Design review of the part built by this model. Coordinates are the model's own, in mm. Give positions to 0.01 mm unless a question says otherwise; leave off trailing zeros. Loops run counter-clockwise (first coordinate to the right, second up) from the corner with the lowest first, then second, coordinate; pieces in that order, holes last. Notation, with made-up numbers: (-20.5, 35.25) -> (-10.5, 35.25) arc R5 ccw to (-10.5, 40.25) -> close; hole circle Ø2 at (37, 73). An arc over 180 degrees is marked (long way). Use a Markdown table: item, result. Add a question column.
1. Draft analysis for pull direction X (two halves, no side actions). For faces 1 (the flat face through (0, 50.2, 2)), 2 (the flat face through (-1.1, -32.5, 0)), state which applies: pulls with the +X half, pulls with the -X half, needs draft (parallel to the pull), parting line crosses it, or undercut.
2. Add section B-B (x = 0). State the section outline as (y, z) points.
3. Add section D-D (x = 36). State the section outline as (y, z) points, and give its area (3 significant figures).
4. Add section C-C (z = 2.75). State the section outline as (x, y) points, and give its area (3 significant figures).
5. For pin 1 Ø1.5 at (y, z) = (62, 3.5) entering from -X; pin 2 Ø1.5 at (x, z) = (-57, 1.5) entering from -Y; pin 3 Ø1.5 at (x, z) = (13, 1.5) entering from +Y, all flat-tipped, find the tip position at first contact; note any pin that passes through.
6. To check wall thickness, follow line 1 (Y direction, x = -0.5, z = 3.95); line 2 (Y direction, x = -24.5, z = 2.35); line 3 (Y direction, x = 6.5, z = 2.2). State the ranges of each line that lie inside material, in increasing order.
7. Add section A-A (y = 0). State the section outline as (x, z) points.
Autodesk Inventor part; units mm, degrees
ref_plane "YZ Plane" through (0, 0, 0) normal (1, 0, 0) x (0, 1, 0)
ref_plane "XZ Plane" through (0, 0, 0) normal (0, 1, 0) x (-1, 0, 0)
ref_plane "XY Plane" through (0, 0, 0) normal (0, 0, 1) x (1, 0, 0)
sketch "Skizze1" plane through (0, 0, 0) normal (0, 0, 1) x (1, 0, 0)
  circle A0 centre (0, 0) radius 80 construction
  circle A1 centre (0, 0) radius 76 construction
  circle A2 centre (0, 0) radius 75.5
  line L0 (-15, 25) -> (15, 25) construction
  line L1 (15, 25) -> (15, -25) construction
  line L2 (15, -25) -> (-15, -25) construction
  line L3 (-15, -25) -> (-15, 25) construction
  line L4 (-15, 25) -> (15, -25) construction
  line L5 (15, 25) -> (-15, -25) construction
  line L6 (-40.1, -27) -> (40.1, -27)
  line L7 (40.1, -27) -> (40.1, -32.2)
  line L8 (40.1, -32.2) -> (-40.1, -32.2)
  line L9 (-40.1, -32.2) -> (-40.1, -27)
  line L10 (-2.6, -32.2) -> (2.6, -32.2)
  line L11 (-30.1, 45) -> (30.1, 45)
  line L12 (30.1, 45) -> (30.1, 50.2)
  line L13 (30.1, 50.2) -> (-30.1, 50.2)
  line L14 (-30.1, 50.2) -> (-30.1, 45)
  line L15 (-2.6, -37.2) -> (2.6, -37.2)
  line L16 (2.6, -37.2) -> (2.6, -62.4)
  line L17 (2.6, -62.4) -> (-2.6, -62.4)
  line L18 (-2.6, -62.4) -> (-2.6, -37.2)
  line L19 (-20, 20) -> (20, 20)
  line L20 (20, 20) -> (20, -20)
  line L21 (20, -20) -> (-20, -20)
  line L22 (-20, -20) -> (-20, 20)
  line L23 (-20, 20) -> (20, -20) construction
  line L24 (20, 20) -> (-20, -20) construction
  line L25 (-2.6, 70.4) -> (2.6, 70.4)
  line L26 (2.6, 70.4) -> (2.6, 55.2)
  line L27 (2.6, 55.2) -> (-2.6, 55.2)
  line L28 (-2.6, 55.2) -> (-2.6, 70.4)
  point P0 (0, -32.2)
  point P1 (0, -32.2)
  point P2 (0, -32.2)
  point P3 (0, 45)
  point P4 (0, -37.2)
  dimension "d0" = 160
  dimension "d1" = 4
  dimension "d2" = 0.5
  dimension "d6" = 30
  dimension "d7" = 50
  dimension "d8" = 2
  dimension "d9" = 80.2
  dimension "d10" = 5.2
  dimension "d13" = 5.2
  dimension "d14" = 60.2
  dimension "d15" = 5.2
  dimension "d16" = 45
  dimension "d17" = 5.2
  dimension "d18" = 25.2
  dimension "d19" = 5
  dimension "d20" = 40
  dimension "d21" = 5
  dimension "d22" = 15.2
extrude "Extrusion1" add sketch "Skizze1" along normal blind 5
properties part number "Slider_1"
Taken from the geometry:
| question | item | result |
|---|---|---|
| 1 | face 1 | undercut |
| 1 | face 2 | needs draft |
| 2 | outline | (-75.5, 0) -> (-62.4, 0) -> (-62.4, 5) -> (-75.5, 5) -> close; (-37.2, 0) -> (-32.2, 0) -> (-32.2, 5) -> (-37.2, 5) -> close; (-27, 0) -> (-20, 0) -> (-20, 5) -> (-27, 5) -> close; (20, 0) -> (45, 0) -> (45, 5) -> (20, 5) -> close; (50.2, 0) -> (55.2, 0) -> (55.2, 5) -> (50.2, 5) -> close; (70.4, 0) -> (75.5, 0) -> (75.5, 5) -> (70.4, 5) -> close |
| 3 | outline | (-66.36, 0) -> (-32.2, 0) -> (-32.2, 5) -> (-66.36, 5) -> close; (-27, 0) -> (66.36, 0) -> (66.36, 5) -> (-27, 5) -> close |
| 3 | area | 638 mm^2 |
| 4 | outline | circle Ø151 at (0, 0); hole (-40.1, -32.2) -> (40.1, -32.2) -> (40.1, -27) -> (-40.1, -27) -> close; hole (-30.1, 45) -> (30.1, 45) -> (30.1, 50.2) -> (-30.1, 50.2) -> close; hole (-20, -20) -> (20, -20) -> (20, 20) -> (-20, 20) -> close; hole (-2.6, -62.4) -> (2.6, -62.4) -> (2.6, -37.2) -> (-2.6, -37.2) -> close; hole (-2.6, 55.2) -> (2.6, 55.2) -> (2.6, 70.4) -> (-2.6, 70.4) -> close |
| 4 | area | 15,400 mm^2 |
| 5 | pin 1 | stops at x = -44.14 |
| 5 | pin 2 | stops at y = -50.36 |
| 5 | pin 3 | stops at y = 74.5 |
| 6 | line 1 | y = -75.5 to -62.4, -37.2 to -32.2, -27 to -20, 20 to 45, 50.2 to 55.2, 70.4 to 75.5 |
| 6 | line 2 | y = -71.41 to -32.2, -27 to 45, 50.2 to 71.41 |
| 6 | line 3 | y = -75.22 to -32.2, -27 to -20, 20 to 45, 50.2 to 75.22 |
| 7 | outline | (-75.5, 0) -> (-20, 0) -> (-20, 5) -> (-75.5, 5) -> close; (20, 0) -> (75.5, 0) -> (75.5, 5) -> (20, 5) -> close |
